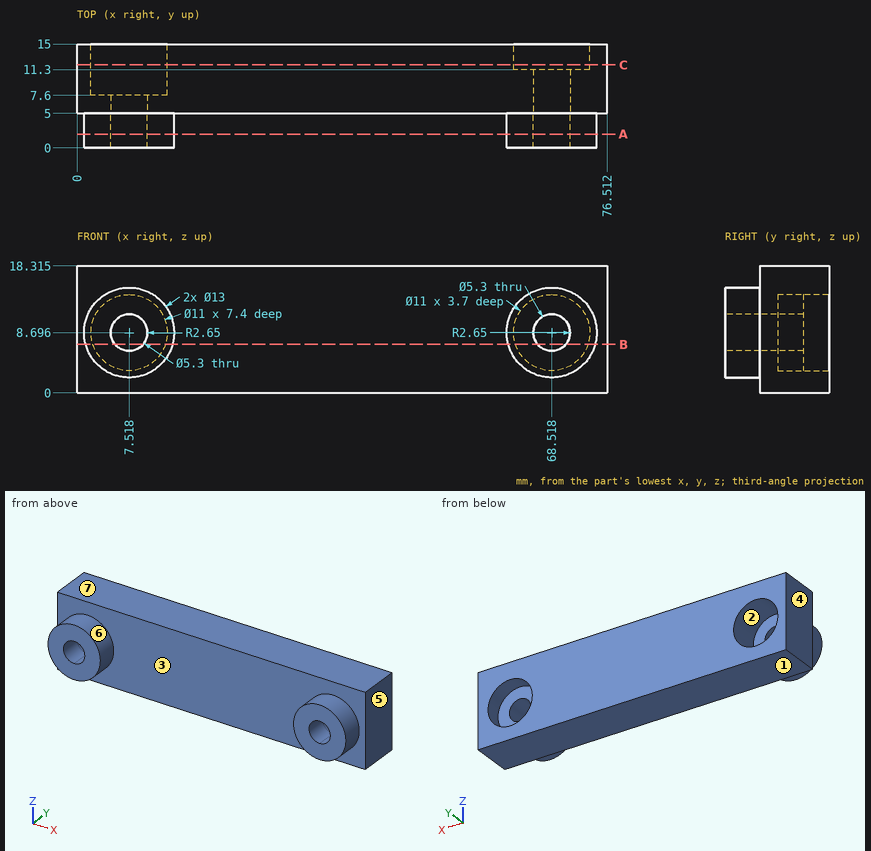
The figure shows three views and two pictorial views of one solid part (mm, origin at its lowest corner). Answer the questions. A direction names the side the tool comes from. Give positions to 0.01 mm unless a question says otherwise; leave off trailing zeros. Write each loop counter-clockwise with the first axis right and the second up, starting at its lowest first coordinate (ties: lowest second). Pieces come first, ordered by that corner, then holes. Notation, with made-up numbers: (76.25, 70.25) -> (116.25, 70.25) arc R8 ccw to (116.25, 75.25) -> close; hole circle Ø6 at (56.25, 89.25). An arc over 180 degrees is marked (long way). Write each question's results on one line, items separated by ' | '.
1. Each of these flat-tipped pins is pushed along its axis until it touches: pin 1 Ø4 at (x, z) = (32, 9) entering from -Y; pin 2 Ø10 at (x, z) = (7.52, 8.7) entering from +Y; pin 3 Ø7 at (x, z) = (68.52, 8.7) entering from +Y. Where does it stop, or does it pass through?
Data:
pin 1: y = 5 | pin 2: y = 7.6 | pin 3: y = 11.3
2. Find section C-C on y = 12. Determine the outline of the cut face in (x, z) (1 decimal).
Data:
outline: (0, 0) -> (76.5, 0) -> (76.5, 18.3) -> (0, 18.3) -> close; hole circle Ø11 at (7.5, 8.7); hole circle Ø11 at (68.5, 8.7)
3. Find section A-A on y = 2. Determine the outline of the cut face in (x, z), and give its area (3 significant figures).
Data:
outline: circle Ø13 at (7.52, 8.7); circle Ø13 at (68.52, 8.7); hole circle Ø5.3 at (7.52, 8.7); hole circle Ø5.3 at (68.52, 8.7) | area: 221 mm^2
4. Straight lines are drawn through the part: L1, parallel to X at y = 12.25, z = 12.5 (1 decimal); L2, parallel to X at y = 13.75, z = 6.5 (1 decimal); L3, parallel to Y at x = 6, z = 16.5. For each, find the intervals that lie inside material, in ascending order.
Data:
L1: 0 to 3.5, 11.5 to 64.5, 72.5 to 76.5 | L2: 0 to 2.5, 12.6 to 63.5, 73.6 to 76.5 | L3: 5 to 15
5. A tool of negligible diameter and unlimited length cuts with its end or side. For the marked faces 1, 2 and 3, from which of +Z, -Z, +X, -X, +Y, -Y can it reach the whole face along a straight path? Write none if from no direction.
Data:
face 1: -Z, +X, -X, +Y, -Y | face 2: +Y | face 3: -Y
6. Find section B-B on z = 7. Give the number of separate pieces and of enclosed holes in the cut face.
Data:
separate pieces: 3 | enclosed holes: 0
7. Determine the mould class of the marked faces 4, 5, 6 and 7 for opening direction X: +X half, -X half, draft (parallel to the pull), parting line (faces both ways), or undercut.
Data:
face 4: -X half | face 5: +X half | face 6: undercut | face 7: draft
